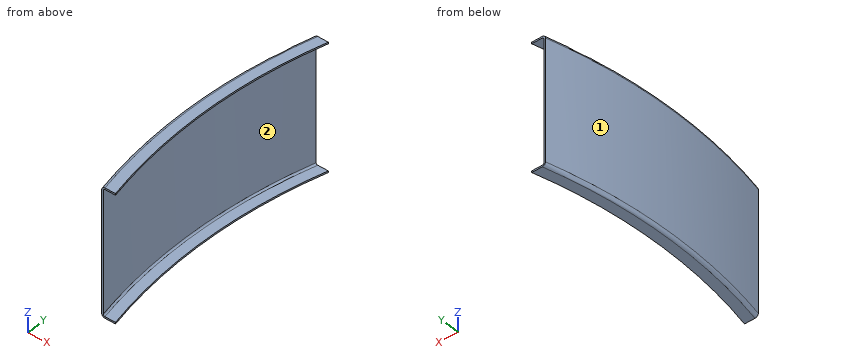
```python
from build123d import *

# Parameters (mm, degrees)
F3_W     = 310
F3_H     = 1324
F4_DEPTH = 100
F5_W     = 1324
F5_H     = 488.598477
F6_DEPTH = 100


with BuildPart() as f2:
    # F2: sweep along a path in F1
    with BuildLine(Plane.XY) as f2_path:
        ThreePointArc((0, 660), (-660, 0), (0, -660))
    # F0 (on Right) → F2 (sweep)
    with BuildSketch(Plane.YZ):
        with BuildLine():
            Line((-658, 77.5), (-645, 77.5))
            Line((-645, 77.5), (-645, 79.5))
            Line((-645, 79.5), (-658, 79.5))
            ThreePointArc((-658, 79.5), (-660.828427, 78.328427), (-662, 75.5))
            Line((-662, 75.5), (-662, -75.5))
            ThreePointArc((-662, -75.5), (-660.828427, -78.328427), (-658, -79.5))
            Line((-658, -79.5), (-645, -79.5))
            Line((-645, -79.5), (-645, -77.5))
            Line((-645, -77.5), (-658, -77.5))
            ThreePointArc((-658, -77.5), (-659.414214, -76.914214), (-660, -75.5))
            Line((-660, -75.5), (-660, 75.5))
            ThreePointArc((-660, 75.5), (-659.414214, 76.914214), (-658, 77.5))
        make_face()
    sweep(path=f2_path.line)

    # F3 (on Top) → F4 (cut, symmetric)
    with BuildSketch(Plane.XY):
        Rectangle(F3_W, F3_H)
    extrude(amount=F4_DEPTH, both=True, mode=Mode.SUBTRACT)

    # F5 (on Top) → F6 (cut, symmetric)
    with BuildSketch(Plane.XY):
        with Locations((0, 399.299239)):
            Rectangle(F5_W, F5_H)
        with Locations((0, -399.299239)):
            Rectangle(F5_W, F5_H)
    extrude(amount=F6_DEPTH, both=True, mode=Mode.SUBTRACT)


solid = f2.part
```
Verification items for the finished model (mm, model axes). Face numbers are marked on the shaded views. A direction names the side the tool comes from. Round coordinates to 2 decimals unless told otherwise and drop trailing zeros. Order: outer loops, then holes, each group sorted by start corner. A loop starts at its lowest first (then second) coordinate and runs counter-clockwise, first axis right, second up. Notation, with made-up numbers: (-3, 25) - (4, 25) arc R17 ccw to (4, 41) - close; hole circle Ø6 at (-4, 30.25). An arc over 180 degrees is marked (long way). Use CSV: the item, a comma, the result in double quotes.
(1) Thickness scan on probe 1 along Z at (x, y) = (-645, -35.5); probe 2 along Z at (x, y) = (-652, 92.5); probe 3 along X at (y, z) = (124, -23.5). Record the ranges inside material, lowest first. Write a range as from..to.
Entries:
probe 1,"-79.5..-77.5, 77.5..79.5"
probe 2,"-79.46..-77.43, 77.43..79.46"
probe 3,"-650.28..-648.25"
(2) Access from +Z, -Z, +X, -X, +Y, -Y to the whole of each face (thin tool, end or side, straight path). Record for the marked faces 1 and 2.
Entries:
face 1,"+Z, -Z, -X"
face 2,"+X"
(3) Section check B-B on z = 50. Record the boundary of the cut face in (x, y), and give its area (3 significant figures).
Entries:
outline,"(-643.6, -155) - (-641.54, -155) arc R660 cw to (-641.54, 155) - (-643.6, 155) arc R662 ccw to start"
area,"626 mm^2"
(4) Gauge pin test, flat end, axial feed: pin 1 Ø4 at (x, y) = (-656.5, 84.5) entering from +Z. Record the tip position at first contact, or that the pin passes through.
Entries:
pin 1,"z = 79.01"
